from build123d import *

# Parameters (mm, degrees)
F1_DEPTH = 40
F2_R     = 5
F3_T     = -1


with BuildPart() as f1:
    # F0 (on Top) → F1 (new body)
    with BuildSketch(Plane.XY):
        with BuildLine():
            ThreePointArc((-1.2863303848, -17.8535710714), (4.2625307585, -9.6824583655), (6.2136696152, 0))
            ThreePointArc((6.2136696152, 0), (4.2625307585, 9.6824583655), (-1.2863303848, 17.8535710714))
            ThreePointArc((-1.2863303848, 17.8535710714), (-8.7863303848, 0), (-1.2863303848, -17.8535710714))
        make_face()
        with BuildLine():
            ThreePointArc((-1.2863303848, 17.8535710714), (4.2625307585, 9.6824583655), (6.2136696152, 0))
            ThreePointArc((6.2136696152, 0), (4.2625307585, -9.6824583655), (-1.2863303848, -17.8535710714))
            ThreePointArc((-1.2863303848, -17.8535710714), (17.6817434111, -24.9568579619), (35.6861864672, -15.6786825802))
            ThreePointArc((35.6861864672, -15.6786825802), (39.7913383009, -8.3122523633), (41.2136696152, 0))
            ThreePointArc((41.2136696152, 0), (25.8961279808, 23.0488611432), (-1.2863303848, 17.8535710714))
        make_face()
        with BuildLine():
            ThreePointArc((-1.2863303848, -17.8535710714), (-8.7863303848, 0), (-1.2863303848, 17.8535710714))
            ThreePointArc((-1.2863303848, 17.8535710714), (-35.8982282908, 18.2258868112), (-37.7066974288, -16.3407377715))
            ThreePointArc((-37.7066974288, -16.3407377715), (-19.8238884715, -24.9784601851), (-1.2863303848, -17.8535710714))
        make_face()
        with BuildLine():
            ThreePointArc((35.6861864672, -15.6786825802), (17.6817434111, -24.9568579619), (-1.2863303848, -17.8535710714))
            ThreePointArc((-1.2863303848, -17.8535710714), (-19.8238884715, -24.9784601851), (-37.7066974288, -16.3407377715))
            Line((-37.7066974288, -16.3407377715), (0, -60))
            Line((0, -60), (35.6861864672, -15.6786825802))
        make_face()
    extrude(amount=F1_DEPTH)

    # F2
    f2_edges = [f1.edges().sort_by_distance(p)[0] for p in [
        (0, -60, 20),
    ]]
    fillet(f2_edges, radius=F2_R)

    # F3
    f3_openings = [f1.faces().sort_by_distance(p)[0] for p in [
        (-1.14081, -8.463934, 40),
    ]]
    offset(amount=F3_T, openings=f3_openings, kind=Kind.INTERSECTION)


solid = f1.part
Can you work these out from the model? Positions are in its coordinate system, mm. A direction names the side the tool comes from. Coordinates: 2 decimals unless noted, no trailing zeros. Loops run counter-clockwise (first coordinate to the right, second up) from the corner with the lowest first, then second, coordinate; pieces in that order, holes last. Notation, with made-up numbers: (13.25, 3) - (27.25, 3) arc R20 cw to (27.25, 29) - close; hole circle Ø9 at (-8.75, 22). An arc over 180 degrees is marked (long way). Put each result on its own line as item: value. Start each with the question number.
Item 1: If we mould it in two halves opening along Y, with no side actions, what happens to faces 1 (the face through (-20.292, -34.974, 20.227)), 2 (the face through (-2, -7, 1)), 3 (the face through (-1.5, 17.6, 40)), 4 (the face through (-0.11, -57.194, 20.28))? For each: +Y half, -Y half, draft (parallel to the pull), parting line (faces both ways), or undercut.
Item 2: Which directions (+Z, -Z, +X, -X, +Y, -Y) give clear straight access to the entire face, cutting with the end or side of a thin tool? Please do faces 5 (the face through (-0.115, -56.195, 20.773)), 6 (the face through (-35.5, 18.59, 19.72)).
Item 3: For pin 1 (8 mm diameter, centred on x = -21, z = 26, fed in from -Y); pin 2 (1.5 mm diameter, centred on x = -3, z = 12, fed in from +Y); pin 3 (1 mm diameter, centred on y = 16.5, z = 19.5, fed in from +X), each with a flat end and sliding along its axis, tell me the tip position at first contact or that it passes through.
Item 4: Suppose I cut it at A-A (z = 31). Please give me the cut outline in (x, y).
Item 5: Suppose I cut it at C-C (x = 23). Please give me the cut outline in (y, z).
Item 6: Suppose I cut it at B-B (y = -42.5). Please give me the cut outline in (x, z).
Item 7: If I drill on line 1 along X through (y, z) = (17, 38.5); line 2 along Y through (x, z) = (-35, 14); line 3 along Z through (x, y) = (-11.5, 9), over which ranges is the centre line in solid material (lowest first)?
Here are the results:
1. face 1: undercut
1. face 2: undercut
1. face 3: draft
1. face 4: -Y half
2. face 5: +Z
2. face 6: +Z, -Z
3. pin 1: y = -40.32
3. pin 2: y = 19.97
3. pin 3: x = 35.42
4. outline: (-37.71, -16.34) - (-3.92, -55.46) arc R5 ccw to (3.76, -55.33) - (35.69, -15.68) arc R25 ccw to (-1.29, 17.85) arc R25 ccw to start; hole (-36.95, -15.69) - (-3.16, -54.81) arc R4 ccw to (2.98, -54.7) - (34.91, -15.05) arc R24 ccw to (-1.29, 16.42) arc R24 ccw to start
5. outline: (-31.43, 0) - (24.06, 0) - (24.06, 40) - (23.02, 40) - (23.02, 1) - (-29.84, 1) - (-29.84, 40) - (-31.43, 40) - close
6. outline: (-15.11, 0) - (14.09, 0) - (14.09, 40) - (12.81, 40) - (12.81, 1) - (-13.79, 1) - (-13.79, 40) - (-15.11, 40) - close
7. line 1: -37.12 to -35.73, -1.85 to -0.73, 33.15 to 34.54
7. line 2: -19.47 to -17.94, 17.7 to 19.03
7. line 3: 0 to 1
